Autodesk Inventor part; units mm, degrees
ref_plane "YZ Plane" through (0, 0, 0) normal (1, 0, 0) x (0, 1, 0)
ref_plane "XZ Plane" through (0, 0, 0) normal (0, 1, 0) x (-1, 0, 0)
ref_plane "XY Plane" through (0, 0, 0) normal (0, 0, 1) x (1, 0, 0)
sketch "Sketch1" plane through (0, 0, 0) normal (0, 1, 0) x (-1, 0, 0)
  circle A0 centre (0, 0) radius 22.55
  circle A1 centre (0, 0) radius 26
  dimension "d0" = 45.1
  dimension "d1" = 52
extrude "Extrusion1" add sketch "Sketch1" along normal blind 15
sketch "Sketch2" plane through (0, 0, 0) normal (0, -1, 0) x (1, 0, 0)
  circle A0 centre (0, 0) radius 26
  circle A1 centre (0, 0) radius 26
extrude "Extrusion2" add sketch "Sketch2" along normal blind 2
fillet "Fillet1" radius 1 1 edges at (22.55, 15, 0)
sketch "Sketch3" plane through (0, 0, 0) normal (0, 1, 0) x (1, 0, 0)
  circle A0 centre (0, 0) radius 23
extrude "Extrusion3" add sketch "Sketch3" along normal blind 5
sketch "Sketch4" plane through (0, 0, 0) normal (1, 0, 0) x (0, 1, 0)
  line L0 (5, 22.55) -> (5, -22.55)
  circle A0 centre (5, 0) radius 2.5
  line L1 (5, -2.5) -> (5, 2.5)
  dimension "d9" = 5
extrude "Extrusion4" cut sketch "Sketch4" against normal through all
pattern_circular "Circular Pattern1" count 6 over 360 about axis through (0, 0, 0) along (0, 1, 0) of "Extrusion4"
fillet "Fillet2" radius 2 1 edges at (-26, -2, 0)
properties part number "Tapacontenedor"
Read the model definition and answer for the solid it produces. Units are mm, in the model's axes. A direction names the side the tool comes from. Round coordinates to 2 decimals unless told otherwise and drop trailing zeros. Write each loop counter-clockwise with the first axis right and the second up, starting at its lowest first coordinate (ties: lowest second). Pieces come first, ordered by that corner, then holes. Notation, with made-up numbers: M 2,-30 L 60,-30 A19 ccw 60,-10 Z; hole C 10,-14 d6. An arc over 180 degrees is marked long. Use a Markdown table: item, result.
1) Straight lines are drawn through the part: line 1 along Z through (x, y) = (0, 8.25); line 2 along Y through (x, z) = (-3, -14); line 3 along Y through (x, z) = (-9.5, 0). For each, find the intervals that lie inside material, in ascending order. Write a range as [from, to].
Answers follow:
| item | result |
|---|---|
| line 1 | z = [-26, -22.55], [22.55, 26] |
| line 2 | y = [-2, 5] |
| line 3 | y = [-2, 2.5] |
2) The part is cut by section A-A (y = 6). Write down the section's boundary in (x, z), plus the area to 3 significant figures.
Answers follow:
| item | result |
|---|---|
| outline | M -25.9,-2.29 A26 ccw -14.93,-21.28 L -13.2,-18.28 A22.55 cw -22.43,-2.29 Z; M -25.9,2.29 L -22.43,2.29 A22.55 cw -13.2,18.28 L -14.93,21.28 A26 ccw Z; M -10.97,-23.57 A26 ccw 10.97,-23.57 L 9.23,-20.57 A22.55 cw -9.23,-20.57 Z; M -10.97,23.57 L -9.23,20.57 A22.55 cw 9.23,20.57 L 10.97,23.57 A26 ccw Z; M 13.2,-18.28 L 14.93,-21.28 A26 ccw 25.9,-2.29 L 22.43,-2.29 A22.55 cw Z; M 13.2,18.28 A22.55 cw 22.43,2.29 L 25.9,2.29 A26 ccw 14.93,21.28 Z |
| area | 431 mm2 |
3) A tool of negligible diameter and unlimited length cuts with its end or side. For faces 4 (the cylindrical face through (-7.9, 2.5, -13.5)), 5 (the flat face through (0, 5, 16)), from which of +Z, -Z, +X, -X, +Y, -Y can it reach the whole face along a straight path? Write none if from no direction.
Answers follow:
| item | result |
|---|---|
| face 4 | none |
| face 5 | +Y |
4) For a pull along Z with two mould halves and no side action, classify faces 1 (the cylindrical face through (15.7, 2.5, -0.1)), 2 (the flat face through (0, -2, 0)), 3 (the cylindrical face through (-7.8, 2.5, 13.7)) as pulls with the +Z half, pulls with the -Z half, needs draft (parallel to the pull), parting line crosses it, or undercut.
Answers follow:
| item | result |
|---|---|
| face 1 | undercut |
| face 2 | needs draft |
| face 3 | undercut |
5) The part is cut by section B-B (y = 13.25). Write down the section's boundary in (x, z).
Answers follow:
| item | result |
|---|---|
| outline | C 0,0 d52; hole C 0,0 d45.1 |
6) Flat-ended cylindrical pins translate along their axes: pin 1 (5.5 mm diameter, centred on x = 0.5, z = -18, fed in from +Y); pin 2 (1 mm diameter, centred on y = 11, z = -10.5, fed in from +X); pin 3 (2 mm diameter, centred on y = 2.5, z = 7.5, fed in from -X). Find the tip coordinate at first contact, or state that the pin passes through.
Answers follow:
| item | result |
|---|---|
| pin 1 | stops at y = 5 |
| pin 2 | stops at x = 24 |
| pin 3 | stops at x = -25.17 |
